The listing builds one solid part. Answer for the finished solid, in the listing's coordinates (mm). A direction names the side the tool comes from. Round coordinates to 2 decimals unless told otherwise and drop trailing zeros. Write each loop counter-clockwise with the first axis right and the second up, starting at its lowest first coordinate (ties: lowest second). Pieces come first, ordered by that corner, then holes. Notation, with made-up numbers: M 40,-36 L 81,-36 A17 cw 81,-5 Z; hole C 48,27 d8. An arc over 180 degrees is marked long. Put each result on its own line as item: value. Start each with the question number.
```python
from build123d import *

# Parameters (mm, degrees)
F1_DEPTH = 6.35
F3_DEPTH = 6.351
F4_W     = 63.5
F4_H     = 3.175
F4_W_2   = 3.175
F4_H_2   = 50.8
F5_DEPTH = 10.16


with BuildPart() as f1:
    # F0 (on Top) → F1 (new body)
    with BuildSketch(Plane.XY):
        with BuildLine():
            ThreePointArc((0, 6.35), (1.859872, 1.859872), (6.35, 0))
            Line((6.35, 0), (69.85, 0))
            ThreePointArc((69.85, 0), (74.340128, 1.859872), (76.2, 6.35))
            Line((76.2, 6.35), (76.2, 57.15))
            ThreePointArc((76.2, 57.15), (74.340128, 61.640128), (69.85, 63.5))
            Line((69.85, 63.5), (6.35, 63.5))
            ThreePointArc((6.35, 63.5), (1.859872, 61.640128), (0, 57.15))
            Line((0, 57.15), (0, 6.35))
        make_face()
    extrude(amount=F1_DEPTH)

    # F2 (on face) → F3 (cut, through all)
    with BuildSketch(Plane.XY.offset(6.35)):
        with BuildLine():
            ThreePointArc((24.13, 31.75), (22.225, 33.655), (20.32, 31.75))
            Line((20.32, 31.75), (22.225, 31.75))
            Line((22.225, 31.75), (24.13, 31.75))
        make_face()
        with BuildLine():
            ThreePointArc((55.88, 31.75), (53.975, 33.655), (52.07, 31.75))
            Line((52.07, 31.75), (53.975, 31.75))
            Line((53.975, 31.75), (55.88, 31.75))
        make_face()
        with BuildLine():
            Line((53.975, 31.75), (52.07, 31.75))
            ThreePointArc((52.07, 31.75), (53.975, 29.845), (55.88, 31.75))
            Line((55.88, 31.75), (53.975, 31.75))
        make_face()
        with BuildLine():
            Line((22.225, 31.75), (20.32, 31.75))
            ThreePointArc((20.32, 31.75), (22.225, 29.845), (24.13, 31.75))
            Line((24.13, 31.75), (22.225, 31.75))
        make_face()
    extrude(amount=-F3_DEPTH, mode=Mode.SUBTRACT)

    # F4 (on face) → F5 (join)
    with BuildSketch(Plane(origin=(0, 0, 0), x_dir=(1, 0, 0), z_dir=(0, 0, -1))):
        with Locations((38.1, 1.5875)):
            Rectangle(F4_W, F4_H)
        with Locations((77.7875, -31.75)):
            Rectangle(F4_W_2, F4_H_2)
        with Locations((38.1, -65.0875)):
            Rectangle(F4_W, F4_H)
    extrude(amount=-F5_DEPTH)


solid = f1.part
```
Item 1: Section A-A (y = 31.75) is taken. Give the vertices of the cut face in (x, z) (3 decimals).
Item 2: Section D-D (y = 55.5) is taken. Give the vertices of the cut face in (x, z) (3 decimals), and give its area (3 significant figures).
Item 3: Flat-ended cylindrical pins translate along their axes: pin 1 (1.9 mm diameter, centred on y = 28.5, z = 7.5, fed in from -X); pin 2 (2.5 mm diameter, centred on x = 77.5, z = 4.5, fed in from +Y); pin 3 (1.6 mm diameter, centred on x = 78.5, z = 3.5, fed in from -Y). Find the tip coordinate at first contact, or state that the pin passes through.
Item 4: Section C-C (x = 30) is taken. Give the vertices of the cut face in (y, z) (3 decimals), and give its area (3 significant figures).
Item 5: Consider line 1 along X through (y, z) = (31.75, 3.75) (3 decimals); line 2 along Y through (x, z) = (64, 9.25) (3 decimals); line 3 along X through (y, z) = (31, 1) (3 decimals). Determine where each line is inside the solid, lowest interval first. Write a range as [from, to].
Item 6: Which of the six approach directions +Z, -Z, +X, -X, +Y, -Y give full straight-line access (tool end or side, diameter ignored) to faces 1 (the flat face through (38, 63.5, 8)), 2 (the flat face through (69.85, -2, 5)), 3 (the flat face through (76.2, 32, 8)), 4 (the flat face through (78, 57.15, 5))?
Item 7: Determine the mould class of faces 5 (the flat face through (38, 0, 8)), 6 (the flat face through (69.85, 65, 5)), 7 (the cylindrical face through (1.91, 61.69, 3.13)) for opening direction Y: released by +Y, released by -Y, zero draft, split by the parting line, or undercut.
Item 8: Section B-B (z = 5.5) is taken. Give the vertices of the cut face in (x, y) (3 decimals).
Output values:
1. outline: M 0,0 L 20.32,0 L 20.32,6.35 L 0,6.35 Z; M 24.13,0 L 52.07,0 L 52.07,6.35 L 24.13,6.35 Z; M 55.88,0 L 79.375,0 L 79.375,10.16 L 76.2,10.16 L 76.2,6.35 L 55.88,6.35 Z
2. outline: M 0,0 L 79.375,0 L 79.375,10.16 L 76.2,10.16 L 76.2,6.35 L 0,6.35 Z
2. area: 516 mm^2
3. pin 1: stops at x = 76.2
3. pin 2: stops at y = 57.15
3. pin 3: stops at y = 6.35
4. outline: M -3.175,0 L 66.675,0 L 66.675,10.16 L 63.5,10.16 L 63.5,6.35 L 0,6.35 L 0,10.16 L -3.175,10.16 Z
4. area: 468 mm^2
5. line 1: x = [0, 20.32], [24.13, 52.07], [55.88, 79.375]
5. line 2: y = [-3.175, 0], [63.5, 66.675]
5. line 3: x = [0, 20.474], [23.976, 52.224], [55.726, 79.375]
6. face 1: +Z, +X, -X
6. face 2: +Z, -Z, +X, -Y
6. face 3: +Z, -X, +Y, -Y
6. face 4: +Z, -Z, +X, +Y
7. face 5: undercut
7. face 6: zero draft
7. face 7: released by +Y
8. outline: M 0,6.35 A6.35 ccw 6.35,0 L 6.35,-3.175 L 69.85,-3.175 L 69.85,0 A6.35 ccw 76.2,6.35 L 79.375,6.35 L 79.375,57.15 L 76.2,57.15 A6.35 ccw 69.85,63.5 L 69.85,66.675 L 6.35,66.675 L 6.35,63.5 A6.35 ccw 0,57.15 Z; hole C 22.225,31.75 d3.81; hole C 53.975,31.75 d3.81
